CAD build for the part. Positions are in the model's coordinates, mm. A direction names the side the tool comes from. Round coordinates to 2 decimals unless told otherwise and drop trailing zeros. Loops run counter-clockwise (first coordinate to the right, second up) from the corner with the lowest first, then second, coordinate; pieces in that order, holes last. Notation, with made-up numbers: (10, -35) - (20, -35) arc R33 cw to (20, -5) - close; hole circle Ø11 at (21.25, 14.5). An arc over 180 degrees is marked (long way). Use one line per item in the form item = value.
from build123d import *

# Parameters (mm, degrees)
SKETCH_1_W           = 7.8
SKETCH_1_H           = 83.4
EXTRUDE_1_DEPTH      = 105
CUT_EXTRUDE_1_DEPTH  = 135.318278726
SKETCH_3_R           = 6
CUT_EXTRUDE_2_DEPTH  = 135.318278726
SKETCH_4_R           = 13.6
CUT_EXTRUDE_3_DEPTH  = 4
SKETCH_5_R           = 1.25
CUT_EXTRUDE_4_DEPTH  = 4
EXTRUDE_2_DEPTH      = 7.2
SKETCH_7_W           = 6
SKETCH_7_H           = 30
CUT_EXTRUDE_5_DEPTH  = 7.2
CUT_EXTRUDE_6_DEPTH  = 135.92798079
SKETCH_9_R           = 1.65
CUT_EXTRUDE_7_DEPTH  = 15
CUT_EXTRUDE_8_DEPTH  = 135.92798079
FILLET_1_R           = 5
CUT_EXTRUDE_10_DEPTH = 135.92798079
SKETCH_16_R          = 1.6
CUT_EXTRUDE_11_DEPTH = 135.92798079
SKETCH_17_R          = 3
CUT_EXTRUDE_12_DEPTH = 2


with BuildPart() as part:
    # 草图1 → 凸台-拉伸1 (new body)
    with BuildSketch(Plane(origin=(0, 0, 0), x_dir=(1, 0, 0), z_dir=(0, 1, 0))):
        with Locations((3.9, -41.7)):
            Rectangle(SKETCH_1_W, SKETCH_1_H)
    extrude(amount=EXTRUDE_1_DEPTH)

    # 草图2 → 切除-拉伸1 (cut, through all)
    with BuildSketch(Plane.ZY):
        with BuildLine():
            Line((0, 64.3), (0, 105))
            Line((0, 105), (32.622555426, 105))
            ThreePointArc((32.622555426, 105), (9.162180169, 90.380266115), (0, 64.3))
        make_face()
        with BuildLine():
            Line((83.4, 105), (83.4, 64.3))
            ThreePointArc((83.4, 64.3), (74.237819831, 90.380266115), (50.777444574, 105))
            Line((50.777444574, 105), (83.4, 105))
        make_face()
    extrude(amount=-CUT_EXTRUDE_1_DEPTH, mode=Mode.SUBTRACT)

    # 草图3 → 切除-拉伸2 (cut, through all)
    with BuildSketch(Plane.ZY):
        with Locations((41.7, 64.3)):
            Circle(SKETCH_3_R)
    extrude(amount=-CUT_EXTRUDE_2_DEPTH, mode=Mode.SUBTRACT)

    # 草图4 → 切除-拉伸3 (cut)
    with BuildSketch(Plane.ZY):
        with Locations((41.7, 64.3)):
            Circle(SKETCH_4_R)
    extrude(amount=-CUT_EXTRUDE_3_DEPTH, mode=Mode.SUBTRACT)

    # 草图5 → 切除-拉伸4 (cut)
    with BuildSketch(Plane.ZY.offset(-4)):
        with Locations((32.2, 64.3)):
            Circle(SKETCH_5_R)
        with Locations((51.2, 64.3)):
            Circle(SKETCH_5_R)
    extrude(amount=-CUT_EXTRUDE_4_DEPTH, mode=Mode.SUBTRACT)

    # 草图6 → 凸台-拉伸2 (add)
    with BuildSketch(Plane(origin=(7.8, 0, 0), x_dir=(0, 0, -1), z_dir=(1, 0, 0))):
        with BuildLine():
            ThreePointArc((-14.146415841, 30), (-26.974511893, 22.286540784), (-41.7, 19.6))
            Line((-41.7, 19.6), (-41.7, 0))
            Line((-41.7, 0), (0, 0))
            Line((0, 0), (0, 30))
            Line((0, 30), (-14.146415841, 30))
        make_face()
        with BuildLine():
            Line((-41.7, 0), (-41.7, 19.6))
            ThreePointArc((-41.7, 19.6), (-56.425488107, 22.286540784), (-69.253584159, 30))
            Line((-69.253584159, 30), (-83.4, 30))
            Line((-83.4, 30), (-83.4, 0))
            Line((-83.4, 0), (-41.7, 0))
        make_face()
    extrude(amount=EXTRUDE_2_DEPTH)

    # 草图7 → 切除-拉伸5 (cut)
    with BuildSketch(Plane(origin=(15, 0, 0), x_dir=(0, 0, -1), z_dir=(1, 0, 0))):
        with Locations((-80.4, 15)):
            Rectangle(SKETCH_7_W, SKETCH_7_H)
    extrude(amount=-CUT_EXTRUDE_5_DEPTH, mode=Mode.SUBTRACT)

    # 草图8 → 切除-拉伸6 (cut, through all)
    with BuildSketch(Plane.ZY):
        with BuildLine():
            Line((31.7, 17), (51.7, 17))
            ThreePointArc((51.7, 17), (55.235533906, 15.535533906), (56.7, 12))
            Line((56.7, 12), (56.7, 0))
            Line((56.7, 0), (26.7, 0))
            Line((26.7, 0), (26.7, 12))
            ThreePointArc((26.7, 12), (28.164466094, 15.535533906), (31.7, 17))
        make_face()
    extrude(amount=-CUT_EXTRUDE_6_DEPTH, mode=Mode.SUBTRACT)

    # 草图9 → 切除-拉伸7 (cut)
    with BuildSketch(Plane.XZ):
        with Locations(Location((7.5, 73.4, 0), (0, 0, 270))):
            Circle(SKETCH_9_R)
        with Locations(Location((7.5, 62.7, 0), (0, 0, 270))):
            Circle(SKETCH_9_R)
        with Locations(Location((7.5, 20.7, 0), (0, 0, 270))):
            Circle(SKETCH_9_R)
        with Locations(Location((7.5, 6, 0), (0, 0, 270))):
            Circle(SKETCH_9_R)
    extrude(amount=-CUT_EXTRUDE_7_DEPTH, mode=Mode.SUBTRACT)

    # 草图10 → 切除-拉伸8 (cut, through all)
    with BuildSketch(Plane.ZY):
        with BuildLine():
            ThreePointArc((71.465786865, 68.759293912), (59.594392775, 88.500786704), (37.240706088, 94.065786865))
            ThreePointArc((37.240706088, 94.065786865), (34.634213135, 90.540706088), (38.159293912, 87.934213135))
            ThreePointArc((38.159293912, 87.934213135), (55.908255091, 83.51556966), (65.334213135, 67.840706088))
            ThreePointArc((65.334213135, 67.840706088), (68.859293912, 65.234213135), (71.465786865, 68.759293912))
        make_face()
    extrude(amount=-CUT_EXTRUDE_8_DEPTH, mode=Mode.SUBTRACT)

    # 圆角1
    fillet_1_edges = [part.edges().sort_by_distance(p)[0] for p in [
        (11.4, 30, 14.146415841),
        (11.4, 30, 69.253584159),
    ]]
    fillet(fillet_1_edges, radius=FILLET_1_R)

    # 草图15 → 切除-拉伸10 (cut, through all)
    with BuildSketch(Plane.ZY):
        with BuildLine():
            ThreePointArc((51.819846568, 27.213416986), (54.551104159, 31.68578749), (56.268755758, 36.63670043))
            ThreePointArc((56.268755758, 36.63670043), (52.521049565, 42.632924099), (46.524825896, 38.885217906))
            ThreePointArc((46.524825896, 38.885217906), (45.508256582, 35.955085758), (43.891798008, 33.308172603))
            ThreePointArc((43.891798008, 33.308172603), (44.80844448, 26.296770514), (51.819846568, 27.213416986))
        make_face()
    extrude(amount=-CUT_EXTRUDE_10_DEPTH, mode=Mode.SUBTRACT)

    # 草图16 → 切除-拉伸11 (cut, through all)
    with BuildSketch(Plane.ZY):
        with Locations((79.9, 7)):
            Circle(SKETCH_16_R)
        with Locations((79.9, 22)):
            Circle(SKETCH_16_R)
    extrude(amount=-CUT_EXTRUDE_11_DEPTH, mode=Mode.SUBTRACT)

    # 草图17 → 切除-拉伸12 (cut)
    with BuildSketch(Plane.ZY):
        with Locations((79.9, 7)):
            Circle(SKETCH_17_R)
        with Locations((79.9, 22)):
            Circle(SKETCH_17_R)
    extrude(amount=-CUT_EXTRUDE_12_DEPTH, mode=Mode.SUBTRACT)


solid = part.part
1) Slice it at A-A (y = 7). Write the cut outline in (x, z), plus the area to 3 significant figures.
Report:
outline = (0, 0) - (15, 0) - (15, 26.7) - (0, 26.7) - close; (0, 56.7) - (15, 56.7) - (15, 77.4) - (7.8, 77.4) - (7.8, 78.3) - (2, 78.3) - (2, 76.9) - (0, 76.9) - close; (0, 82.9) - (2, 82.9) - (2, 81.5) - (7.8, 81.5) - (7.8, 83.4) - (0, 83.4) - close; hole circle Ø3.3 at (7.5, 6); hole circle Ø3.3 at (7.5, 20.7); hole circle Ø3.3 at (7.5, 62.7); hole circle Ø3.3 at (7.5, 73.4)
area = 693 mm^2
2) Slice it at C-C (z = 62.7). Write the cut outline in (x, y), plus the area to 3 significant figures.
Report:
outline = (0, 0) - (5.85, 0) - (5.85, 15) - (9.15, 15) - (9.15, 0) - (15, 0) - (15, 25.27) - (7.8, 25.27) - (7.8, 75.71) - (0, 75.71) - close; (0, 85.86) - (7.8, 85.86) - (7.8, 100.33) - (0, 100.33) - close
area = 836 mm^2
3) Slice it at D-D (x = 10.75). Write the cut outline in (y, z), plus the area to 3 significant figures.
Report:
outline = (0, 0) - (30, 0) - (30, 12.32) arc R5 ccw to (28.89, 15.47) arc R41.7 cw to (28.89, 67.93) arc R5 ccw to (30, 71.08) - (30, 77.4) - (0, 77.4) - (0, 56.7) - (12, 56.7) arc R5 cw to (17, 51.7) - (17, 31.7) arc R5 cw to (12, 26.7) - (0, 26.7) - close
area = 1,430 mm^2
4) Drill centre lines: probe 1 along Y at (x, z) = (5.2, 41.7); probe 2 along Y at (x, z) = (6.5, 48.5); probe 3 along X at (y, z) = (9, 6). Where is each one in solid material? Low to high.
Report:
probe_1 = 17 to 58.3, 70.3 to 88.2, 94.4 to 105
probe_2 = 17 to 25.3, 41.84 to 87.21, 93.62 to 105
probe_3 = 0 to 5.85, 9.15 to 15
5) Slice it at B-B (y = 22). Write the cut outline in (x, z).
Report:
outline = (0, 0) - (15, 0) - (15, 27.76) - (7.8, 27.76) - (7.8, 55.64) - (15, 55.64) - (15, 77.4) - (7.8, 77.4) - (7.8, 78.3) - (2, 78.3) - (2, 76.9) - (0, 76.9) - close; (0, 82.9) - (2, 82.9) - (2, 81.5) - (7.8, 81.5) - (7.8, 83.4) - (0, 83.4) - close
6) Tool access for faces 4 (the flat face through (2, 20.7, 81.2)), 5 (the cylindrical face through (11.45, 29.705, 69.389)), 6 (the flat face through (8, 15, 63)), 7 (the cylindrical face through (3.85, 83.67, 55.7)): list every direction of +Z, -Z, +X, -X, +Y, -Y with a clear straight run to the whole face (end or side of a thin tool).
Report:
face_4 = -X
face_5 = +X, +Y
face_6 = -Y
face_7 = +X, -X
7) Two-plate mould, pull along Z, no slides. Class faces 1 (the flat face through (11, 15, 77.4)), 2 (the cylindrical face through (5.87, 63.54, 50.21)), 3 (the flat face through (11, 30, 6)): +Z half, -Z half, draft (parallel to the pull), parting line (faces both ways), or undercut.
Report:
face_1 = +Z half
face_2 = undercut
face_3 = draft
8) Flat gauge pins, fed straight in: pin 1 (2 mm diameter, centred on y = 72, z = 11, fed in from -X); pin 2 (3 mm diameter, centred on y = 64.3, z = 51.2, fed in from +X); pin 3 (8 mm diameter, centred on x = 12, z = 3.5, fed in from +Y); pin 4 (8 mm diameter, centred on x = 12, y = 21, fed in from +Z). Where does each tip first touch, or does it go through?
Report:
pin_1 = 0
pin_2 = 7.8
pin_3 = 30
pin_4 = 77.4
